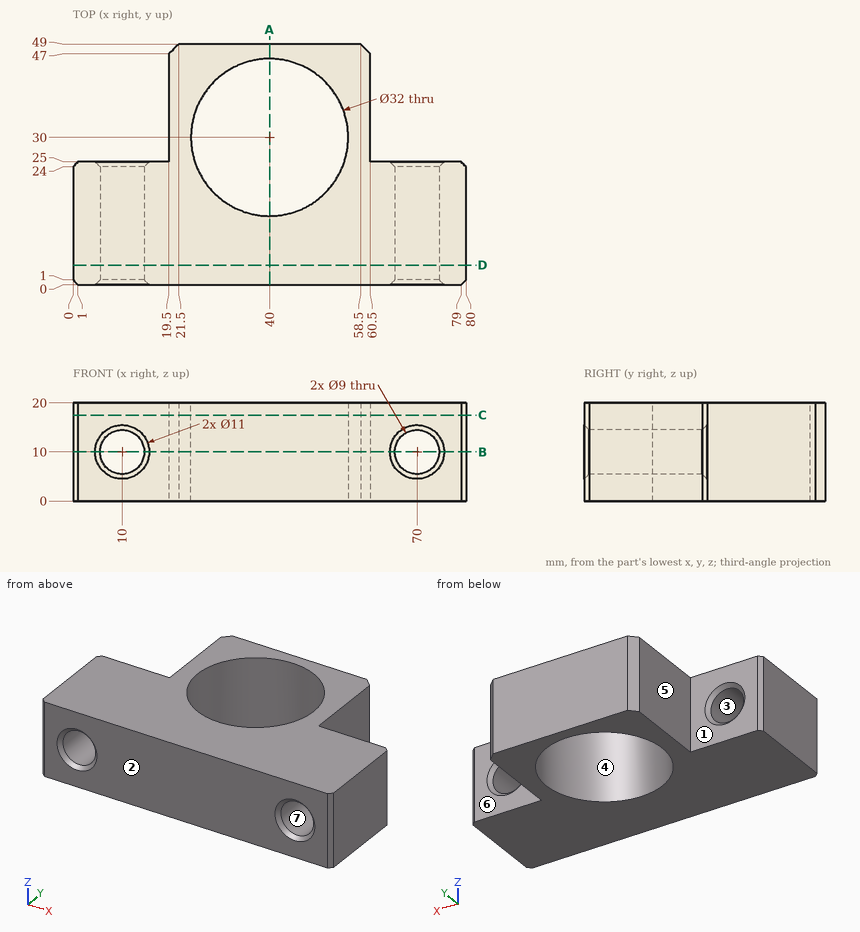
Verification items for this drawing (mm, ordinates from the low corner). A direction names the side the tool comes from. Coordinates: 2 decimals unless noted, no trailing zeros. Order: outer loops, then holes, each group sorted by start corner. A loop starts at its lowest first (then second) coordinate and runs counter-clockwise, first axis right, second up. Notation, with made-up numbers: (45, 42.25) - (57, 42.25) arc R20 ccw to (57, 76.25) - close; hole circle Ø10 at (48, 6.25). An arc over 180 degrees is marked (long way). Answer in a Markdown table with one row per item. Add a question column.
1. Access from +Z, -Z, +X, -X, +Y, -Y to the whole of each face (thin tool, end or side, straight path). Record for the marked faces 5, 6 and 7.
2. Section check C-C (z = 17.5). Enter the section's corners in (x, y).
3. Material ranges on L1, parallel to X at y = 9.5, z = 10; L2, parallel to Y at x = 40, z = 11; L3, parallel to X at y = 17, z = 10, recorded low to high. Write a range as [from, to].
4. Section check A-A (x = 40). Enter the section's corners in (y, z), plus the area to 3 significant figures.
5. Section check B-B (z = 10). Give the number of separate pieces and of enclosed holes in the cut face, plus the area to 3 significant figures.
6. Draft check along Y on the marked faces 1, 2, 3 and 4. Enter one of: +Y half, -Y half, draft (parallel to the pull), parting line (faces both ways), or undercut.
7. Section check D-D (y = 4). Enter the section's corners in (x, z), plus the area to 3 significant figures.
8. Gauge pin test, flat ends, axial feed: pin 1 Ø1.5 at (y, z) = (42, 15.5) entering from +X; pin 2 Ø3 at (x, z) = (20.5, 4.5) entering from +Y; pin 3 Ø11.5 at (x, z) = (10, 10) entering from +Y; pin 4 Ø5 at (y, z) = (31.5, 13) entering from -X. Record the tip position at first contact, or that the pin passes through.
Data:
| question | item | result |
|---|---|---|
| 1 | face 5 | +Z, -Z, -X, +Y |
| 1 | face 6 | +Z, -Z, +X, +Y |
| 1 | face 7 | +Y, -Y |
| 2 | outline | (0, 1) - (1, 0) - (79, 0) - (80, 1) - (80, 24) - (79, 25) - (60.5, 25) - (60.5, 47) - (58.5, 49) - (21.5, 49) - (19.5, 47) - (19.5, 25) - (1, 25) - (0, 24) - close; hole circle Ø32 at (40, 30) |
| 3 | L1 | x = [0, 5.5], [14.5, 65.5], [74.5, 80] |
| 3 | L2 | y = [0, 14], [46, 49] |
| 3 | L3 | x = [0, 5.5], [14.5, 30.67], [49.33, 65.5], [74.5, 80] |
| 4 | outline | (0, 0) - (14, 0) - (14, 20) - (0, 20) - close; (46, 0) - (49, 0) - (49, 20) - (46, 20) - close |
| 4 | area | 340 mm² |
| 5 | separate pieces | 3 |
| 5 | enclosed holes | 1 |
| 5 | area | 1,720 mm² |
| 6 | face 1 | +Y half |
| 6 | face 2 | -Y half |
| 6 | face 3 | draft |
| 6 | face 4 | undercut |
| 7 | outline | (0, 0) - (80, 0) - (80, 20) - (0, 20) - close; hole circle Ø9 at (10, 10); hole circle Ø9 at (70, 10) |
| 7 | area | 1,470 mm² |
| 8 | pin 1 | stops at x = 60.5 |
| 8 | pin 2 | stops at y = 49 |
| 8 | pin 3 | stops at y = 25 |
| 8 | pin 4 | stops at x = 19.5 |
